Autodesk Inventor part; units mm, degrees
ref_plane "YZ Plane" through (0, 0, 0) normal (1, 0, 0) x (0, 1, 0)
ref_plane "XZ Plane" through (0, 0, 0) normal (0, 1, 0) x (-1, 0, 0)
ref_plane "XY Plane" through (0, 0, 0) normal (0, 0, 1) x (1, 0, 0)
sketch "Sketch1" plane through (0, 0, 0) normal (0, 1, 0) x (-1, 0, 0)
  line L0 (25.4, 34.925) -> (-25.4, 34.925)
  line L1 (-25.4, 34.925) -> (-25.4, -34.925)
  line L2 (-25.4, -34.925) -> (25.4, -34.925)
  line L3 (25.4, -34.925) -> (25.4, 34.925)
  line L4 (25.4, 34.925) -> (-25.4, -34.925) construction
  line L5 (-25.4, 34.925) -> (25.4, -34.925) construction
  line L6 (25.4, -34.925) -> (12.7, -34.925)
  line L7 (25.4, -22.225) -> (25.4, -34.925)
  line L8 (-25.4, -34.925) -> (-12.7, -34.925)
  line L9 (-12.7, -22.225) -> (-25.4, -22.225)
  line L10 (-25.4, -22.225) -> (-25.4, -34.925)
  line L11 (12.7, -22.225) -> (12.7, 3.175)
  line L12 (12.7, -22.225) -> (38.1, -22.225) construction
  line L13 (-12.7, -22.225) -> (-12.7, 3.175)
  line L14 (25.4, 34.925) -> (12.7, 34.925)
  line L15 (25.4, 22.225) -> (25.4, 34.925)
  line L16 (-25.4, 34.925) -> (-12.7, 34.925)
  line L17 (-25.4, 22.225) -> (-25.4, 34.925)
  circle A0 centre (12.7, 22.225) radius 2.54
  circle A1 centre (-12.7, 22.225) radius 2.54
  circle A2 centre (12.7, -22.225) radius 3.175
  circle A3 centre (-12.7, -22.225) radius 3.175
  circle A4 centre (12.7, 3.175) radius 3.175
  circle A5 centre (-12.7, 3.175) radius 3.175
  point P0 (0, 0)
  dimension "d0" = 50.8
  dimension "d1" = 69.85
  dimension "d2" = 12.7
  dimension "d3" = 12.7
  dimension "d4" = 12.7
  dimension "d5" = 12.7
  dimension "d6" = 25.4
  dimension "d7" = 90
  dimension "d8" = 25.4
  dimension "d13" = 5.08
  dimension "d14" = 5.08
  dimension "d15" = 6.35
  dimension "d16" = 6.35
  dimension "d17" = 6.35
  dimension "d18" = 6.35
extrude "Extrusion1" add sketch "Sketch1" along normal blind 6.35
properties part number "CatapultPlate"
Part model, mm, in its own coordinate system. Round coordinates to 2 decimals unless told otherwise and drop trailing zeros. Write each loop counter-clockwise with the first axis right and the second up, starting at its lowest first coordinate (ties: lowest second). Pieces come first, ordered by that corner, then holes. Notation, with made-up numbers: (37, 58) - (69, 58) arc R12 ccw to (69, 64) - close; hole circle Ø3 at (29, 81). An arc over 180 degrees is marked (long way). Use CSV: the item, a comma, the result in double quotes.
Item 1: Slice it at C-C, the plane x = 13. Write the cut outline in (y, z) (3 decimals), then the cut area to 3 significant figures.
Results list:
outline,"(0, -34.925) - (6.35, -34.925) - (6.35, -25.386) - (0, -25.386) - close; (0, -19.064) - (6.35, -19.064) - (6.35, 0.014) - (0, 0.014) - close; (0, 6.336) - (6.35, 6.336) - (6.35, 19.703) - (0, 19.703) - close; (0, 24.747) - (6.35, 24.747) - (6.35, 34.925) - (0, 34.925) - close"
area,"331 mm²"
Item 2: Flat gauge pin, fed straight in: P1, Ø5.5, axis at x = 12.7, z = -22.225, coming from the -Y side. Where does the tip first touch, or does it go through?
Results list:
P1,"passes through"
Item 3: Slice it at B-B, the plane y = 5.5. Write the cut outline in (x, z) (3 decimals).
Results list:
outline,"(-25.4, -34.925) - (25.4, -34.925) - (25.4, 34.925) - (-25.4, 34.925) - close; hole circle Ø6.35 at (-12.7, -22.225); hole circle Ø6.35 at (-12.7, 3.175); hole circle Ø5.08 at (-12.7, 22.225); hole circle Ø6.35 at (12.7, -22.225); hole circle Ø6.35 at (12.7, 3.175); hole circle Ø5.08 at (12.7, 22.225)"
Item 4: Wall check: L1, parallel to Z at x = -12.7, y = 4.75 (3 decimals); L2, parallel to Z at x = -11, y = 4.25 (3 decimals); L3, parallel to X at y = 4.25, z = 6. Give the ranges that are in metal, low to high.
Results list:
L1,"z = -34.925 to -25.4, -19.05 to 0, 6.35 to 19.685, 24.765 to 34.925"
L2,"z = -34.925 to -24.907, -19.543 to 0.493, 5.857 to 20.338, 24.112 to 34.925"
L3,"x = -25.4 to -14.15, -11.25 to 11.25, 14.15 to 25.4"
Item 5: Pull direction X, two halves, no side cores. Call faces 1 (the flat face through (-25.4, 3, 0)), 2 (the cylindrical face through (-10.18, 3.131, 5.107)), 3 (the cylindrical face through (-10.36, 3.13, -24.37)), 4 (the flat face through (0, 6.35, 0)): pulls with the +X half, pulls with the -X half, needs draft (parallel to the pull), parting line crosses it, or undercut.
Results list:
face 1,"pulls with the -X half"
face 2,"undercut"
face 3,"undercut"
face 4,"needs draft"
Item 6: Slice it at A-A, the plane x = -12.7. Write the cut outline in (y, z) (3 decimals).
Results list:
outline,"(0, -34.925) - (6.35, -34.925) - (6.35, -25.4) - (0, -25.4) - close; (0, -19.05) - (6.35, -19.05) - (6.35, 0) - (0, 0) - close; (0, 6.35) - (6.35, 6.35) - (6.35, 19.685) - (0, 19.685) - close; (0, 24.765) - (6.35, 24.765) - (6.35, 34.925) - (0, 34.925) - close"
